Source: CAD feature listing. Evaluate the final solid. Frame: model axes, mm. Face numbers are marked on the shaded views. A direction names the side the tool comes from. Coordinates: 2 decimals unless noted, no trailing zeros. Loops run counter-clockwise (first coordinate to the right, second up) from the corner with the lowest first, then second, coordinate; pieces in that order, holes last.
Item 1: Reachability of the marked faces 1 and 2 from +Z, -Z, +X, -X, +Y, -Y: full face, straight path, thin tool, end or side. Return the list, or none.
Item 2: Section query B-B, the plane x = 25.5. Return the cut outline in (y, z) (3 decimals), then the cut area to 3 significant figures.
Item 3: Section query C-C, the plane z = -6.5. Return the cut outline in (x, y), then the cut area to 3 significant figures.
Item 4: Line query: probe 1 along Y at (x, z) = (11.43, 1.15); probe 2 along Y at (x, z) = (19.05, 2.4); probe 3 along Z at (x, y) = (13.5, 177.5) (3 decimals). Output: solid intervals per line, ascending.
Item 5: Pin query (flat end, axial travel): pin 1 Ø2 at (y, z) = (52.5, -2) entering from -X; pin 2 Ø1.5 at (y, z) = (75, -5.5) entering from -X; pin 3 Ø3.5 at (x, y) = (11.43, 2.54) entering from +Z; pin 4 Ø1.5 at (y, z) = (128.5, -7.5) entering from +X. Return the tip coordinate at first contact, or that it passes through.
Autodesk Inventor part; units mm, degrees
ref_plane "Work Plane1" through (0, 0, 0) normal (0, 0, 1) x (1, 0, 0)
ref_plane "YZ Plane" through (0, 0, 0) normal (1, 0, 0) x (0, 1, 0)
ref_plane "XZ Plane" through (0, 0, 0) normal (0, 1, 0) x (-1, 0, 0)
ref_plane "Work Plane1" through (0, 0, 0) normal (0, 0, 1) x (1, 0, 0)
sketch "Sketch1" plane through (0, 0, 0) normal (0, 0, 1) x (1, 0, 0)
  circle A0 centre (11.43, 2.54) radius 2.286
  circle A1 centre (19.05, 7.62) radius 2.286
  circle A2 centre (19.05, 252.2398) radius 2.286
  circle A3 centre (11.43, 257.3198) radius 2.286
  line L0 (22.225, -12.7) -> (-22.225, -12.7)
  line L1 (22.225, 272.5598) -> (-22.225, 272.5598)
  line L2 (34.925, -12.7) -> (-22.225, -12.7)
  line L3 (-22.225, -12.7) -> (-22.225, 272.5598) construction
  line L4 (-22.225, 272.5598) -> (34.925, 272.5598)
  line L5 (34.925, 272.5598) -> (34.925, -12.7)
  line L6 (0, 272.5598) -> (0, -12.7)
  point P0 (0, 0)
  point P1 (-22.225, -12.7)
  point P2 (0, -12.7)
  point P3 (0, -12.7)
  dimension "d0" = 57.15
  dimension "d9" = 34.925
extrude "Extrusion1" add sketch "Sketch1" along normal blind 3.175
sketch "Sketch2" plane through (-22.225, 272.5598, 0) normal (0, 1, 0) x (1, 0, 0)
  line L0 (69.8754, 18.7905) -> (57.15, -1.5875) construction
  line L1 (57.15, 0) -> (57.15, -3.175)
  line L2 (66.9043, 17.0297) -> (55.5406, -1.1676)
  line L3 (69.5973, 15.348) -> (58.7765, -1.98)
  arc A0 (57.15, -3.175) -> (58.7765, -1.98) centre (56.4627, -0.5351) ccw
  line L4 (57.15, -3.175) -> (55.5406, -1.1676)
  line L5 (69.5973, 15.348) -> (66.9043, 17.0297)
  point P0 (22.225, 0)
  dimension "d4" = 1.5875
  dimension "d5" = 1.5875
extrude "Extrusion2" add sketch "Sketch2" against normal up to surface (285.2598 mm away)
fillet "Fillet1" radius 6.35 3 edges at (46.0258, 272.5598, -16.1889) (34.0447, 129.9299, 0) (46.0258, -12.7, -16.1889)
properties part number "PolyIntakeTop" material "Polycarbonate, Smoke"
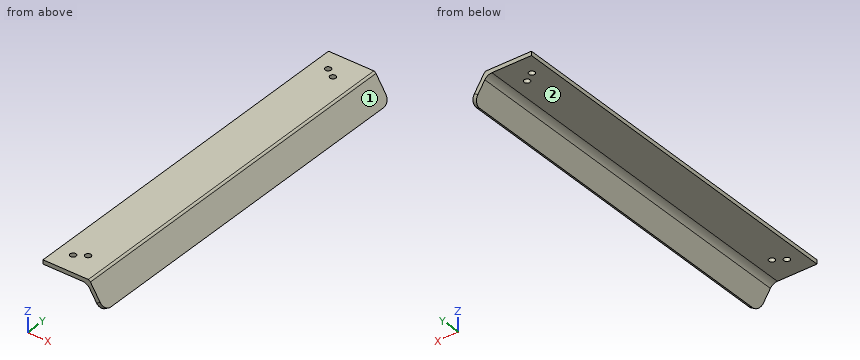
Verdict:
1. face 1: +Z, +X, +Y, -Y
1. face 2: -Z, -X, +Y, -Y
2. outline: (-12.7, 0) - (272.56, 0) - (272.56, 3.175) - (-12.7, 3.175) - close
2. area: 906 mm2
3. outline: (38.1, -12.7) - (41.85, -12.7) - (41.85, 272.56) - (38.1, 272.56) - close
3. area: 1,070 mm2
4. probe 1: y = -12.7 to 0.25, 4.83 to 255.03, 259.61 to 272.56
4. probe 2: y = -12.7 to 5.33, 9.91 to 249.95, 254.53 to 272.56
4. probe 3: z = 0 to 3.175
5. pin 1: stops at x = 33.94
5. pin 2: stops at x = 37.01
5. pin 3: passes through
5. pin 4: stops at x = 42.94
